```python
from build123d import *

# Parameters (mm, degrees)
F1_DEPTH = 12.7


with BuildPart() as f1:
    # F0 (on Front) → F1 (new body)
    with BuildSketch(Plane.XZ):
        with BuildLine():
            Line((148.936364, 23.661141), (27.709091, 70.983423))
            ThreePointArc((27.709091, 70.983423), (-76.2, 0), (27.709091, -70.983423))
            Line((27.709091, -70.983423), (148.936364, -23.661141))
            ThreePointArc((148.936364, -23.661141), (165.1, 0), (148.936364, 23.661141))
        make_face()
        with BuildLine():
            Line((147.781818, -20.703498), (26.554545, -68.02578))
            ThreePointArc((26.554545, -68.02578), (-73.025, 0), (26.554545, 68.02578))
            Line((26.554545, 68.02578), (147.781818, 20.703498))
            ThreePointArc((147.781818, 20.703498), (161.925, 0), (147.781818, -20.703498))
        make_face(mode=Mode.SUBTRACT)
    extrude(amount=F1_DEPTH)


solid = f1.part
```
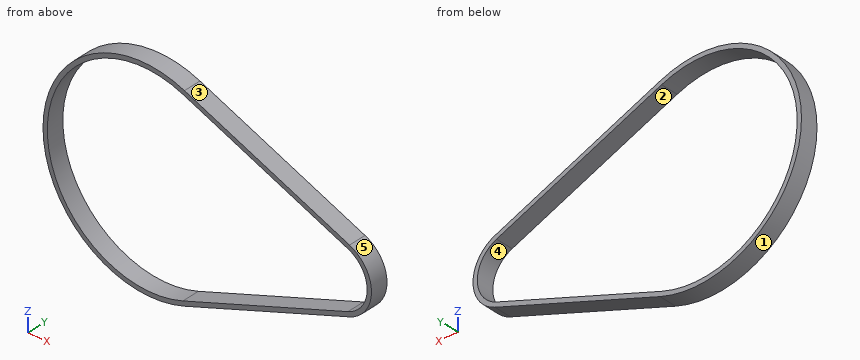
Geometry: final body of the model. Coordinates: model frame, mm. Face numbers are marked on the shaded views. A direction names the side the tool comes from. Round coordinates to 2 decimals unless told otherwise and drop trailing zeros. Write each loop counter-clockwise with the first axis right and the second up, starting at its lowest first coordinate (ties: lowest second). Pieces come first, ordered by that corner, then holes. Notation, with made-up numbers: (26.25, 53.25) -> (85.25, 53.25) arc R23 cw to (85.25, 78.25) -> close; hole circle Ø2 at (20, -14.75). An arc over 180 degrees is marked (long way). Return JSON: item names as keys, results as strings.
Q1. Section C-C on x = 0. Return the cut outline in (y, z) (3 decimals).
From the geometry:
{"outline": "(-12.7, -76.2) -> (0, -76.2) -> (0, -73.025) -> (-12.7, -73.025) -> close; (-12.7, 73.025) -> (0, 73.025) -> (0, 76.2) -> (-12.7, 76.2) -> close"}
Q2. Mould query, pull axis Z, two halves, no side actions, for the marked faces 1, 2 and 3. Classes: +Z half, -Z half, draft (parallel to the pull), parting line (faces both ways), or undercut.
From the geometry:
{"face 1": "parting line", "face 2": "undercut", "face 3": "+Z half"}
Q3. First-contact query: pin 1 Ø5 at (x, y) = (61.5, -3.5) entering from -Z; pin 2 Ø4 at (y, z) = (-8, -12.5) entering from -X; pin 3 Ø2 at (y, z) = (-4, 59.5) entering from -X. Flat tips, straight axial feed; report the tip coordinate or a pass-through.
From the geometry:
{"pin 1": "z = -58.77", "pin 2": "x = -75.47", "pin 3": "x = -48.83"}
Q4. Ray query, line 1 (Z direction, x = 0, y = -9.5) (3 decimals); line 2 (X direction, y = -9.75, z = 0) (3 decimals); line 3 (Z direction, x = 25, y = -0.75). Return the intervals inside material, ascending.
From the geometry:
{"line 1": "-76.2 to -73.025, 73.025 to 76.2", "line 2": "-76.2 to -73.025, 161.925 to 165.1", "line 3": "-71.98 to -68.61, 68.61 to 71.98"}
Q5. Section A-A on z = 0. Return the cut outline in (x, y) (3 decimals).
From the geometry:
{"outline": "(-76.2, -12.7) -> (-73.025, -12.7) -> (-73.025, 0) -> (-76.2, 0) -> close; (161.925, -12.7) -> (165.1, -12.7) -> (165.1, 0) -> (161.925, 0) -> close"}
Q6. Set-up query: the marked faces 4 and 5. Return all of +Z, -Z, +X, -X, +Y, -Y with unobstructed straight access to the full face (end or side cutting, diameter ignored); none if empty.
From the geometry:
{"face 4": "+Y, -Y", "face 5": "+X, +Y, -Y"}
